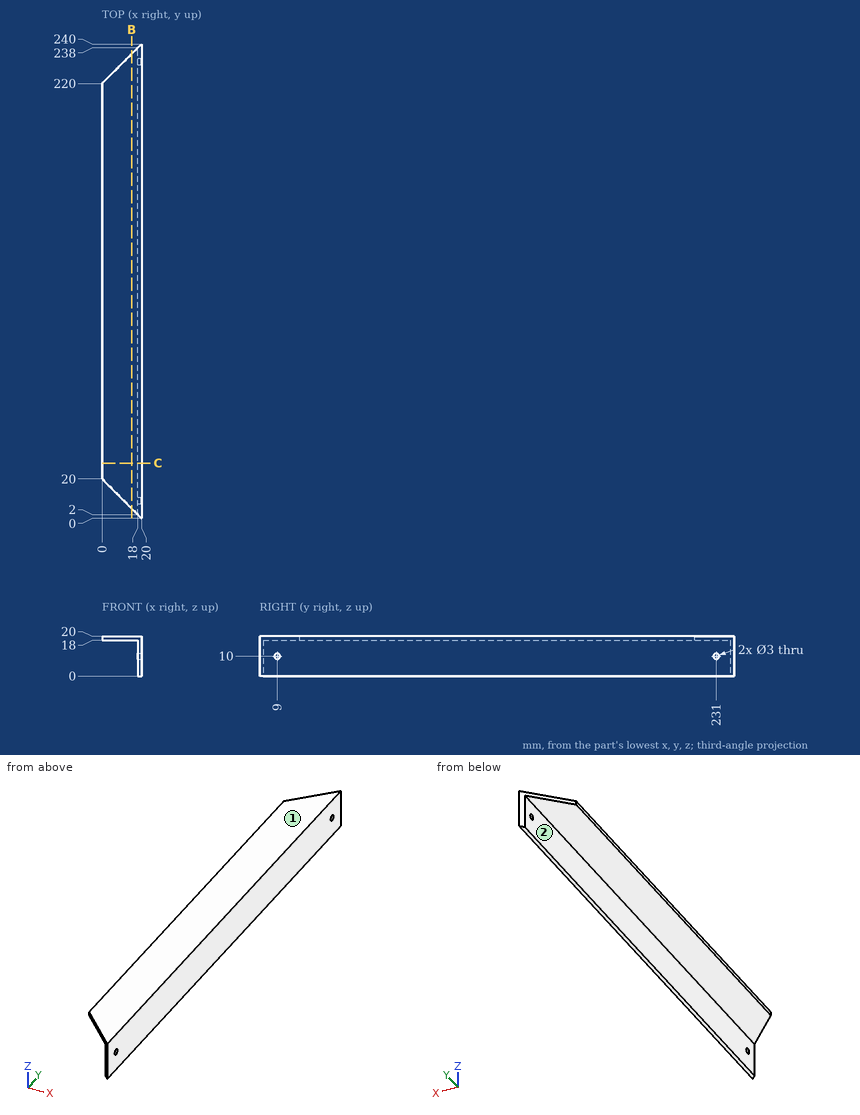
Print and shaded views of the part. All mm, measured from the part's lowest x, y and z. A direction names the side the tool comes from. Coordinates: 2 decimals unless noted, no trailing zeros. Order: outer loops, then holes, each group sorted by start corner. A loop starts at its lowest first (then second) coordinate and runs counter-clockwise, first axis right, second up. Notation, with made-up numbers: (69.5, -24) - (98.5, -24) arc R33 ccw to (98.5, 6) - close; hole circle Ø3 at (-6.5, 23). An arc over 180 degrees is marked (long way). Return JSON: item names as keys, results as strings. Group by question number.
Item 1: Which spindle directions (+Z, -Z, +X, -X, +Y, -Y) get a long thin tool onto all of the face, cutting with end or side? Do the marked faces 1 and 2. Say none if no direction does.
Item 2: Cut at B-B (x = 15). List the corners of the cut face in (y, z), plus the area to 3 significant figures.
Item 3: Cut at C-C (y = 28). List the corners of the cut face in (x, z), plus the area to 3 significant figures.
Item 4: Pin check, flat tips, straight feed: pin 1 (10 mm diameter, centred on x = 12.5, z = 11.5, fed in from +Y); pin 2 (4 mm diameter, centred on x = 5, y = 176.5, fed in from -Z); pin 3 (9 mm diameter, centred on y = 146.5, z = 8.5, fed in from -X). Stop position of each tip, or through.
Item 5: Drill centre lines: probe 1 along Z at (x, y) = (19.1, 9); probe 2 along X at (y, z) = (168.5, 10.75). Where is each one in solid material? Low to high. Write a range as from..to.
Check values:
{
 "1": {"face 1": "+Z, +X, -X, +Y, -Y", "face 2": "-Z, -X, +Y, -Y"},
 "2": {"outline": "(5, 18) - (235, 18) - (235, 20) - (5, 20) - close", "area": "460 mm2"},
 "3": {"outline": "(0, 18) - (18, 18) - (18, 0) - (20, 0) - (20, 20) - (0, 20) - close", "area": "76.0 mm2"},
 "4": {"pin 1": "passes through", "pin 2": "stops at z = 18", "pin 3": "stops at x = 18"},
 "5": {"probe 1": "z = 0..8.5, 11.5..20", "probe 2": "x = 18..20"}
}
